from build123d import *

# Parameters (mm, degrees)
SKETCH1_R                         = 4
EXTRUDE1_DEPTH                    = 400
SKETCH3_W                         = 2
SKETCH3_H                         = 4
F_4_0_4_DIAMETER_HOLE1_AT_2_COUNT = 2
F_4_0_4_DIAMETER_HOLE1_AT_2_PITCH = 380


with BuildPart() as part:
    # Sketch1 → Extrude1 (new body)
    with BuildSketch(Plane.XY):
        Circle(SKETCH1_R)
    extrude(amount=EXTRUDE1_DEPTH)

    # Sketch3 → Ø4.0 (4) Diameter Hole1 (revolve, cut)
    with BuildSketch(Plane(origin=(0, 0, 10), x_dir=(0, 0, -1), z_dir=(1, 0, 0))):
        with Locations((1, 2)):
            Rectangle(SKETCH3_W, SKETCH3_H)
    f_4_0_4_diameter_hole1 = revolve(axis=Axis((0, -6.35, 10), (0, 1, 0)), mode=Mode.SUBTRACT)

    # Ø4.0 (4) Diameter Hole1 at 2: Ø4.0 (4) Diameter Hole1 ×2
    with Locations(*[(0, 0, i * F_4_0_4_DIAMETER_HOLE1_AT_2_PITCH) for i in range(1, F_4_0_4_DIAMETER_HOLE1_AT_2_COUNT)]):
        add(f_4_0_4_diameter_hole1, mode=Mode.SUBTRACT)


solid = part.part
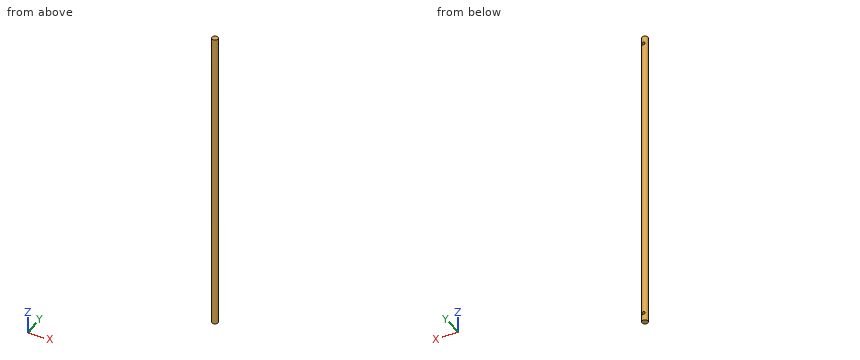
Work out the finished part from the listing and answer in its coordinate system (mm). Give positions to 0.01 mm unless a question says otherwise; leave off trailing zeros. Order: outer loops, then holes, each group sorted by start corner. A loop starts at its lowest first (then second) coordinate and runs counter-clockwise, first axis right, second up. Notation, with made-up numbers: (8, 30.25) -> (21, 30.25) arc R19 ccw to (21, 51.25) -> close; hole circle Ø6 at (-33.5, 59.5). An arc over 180 degrees is marked (long way). Answer as a JSON object with one key per item and string values. Group by question number.
1. Flat-ended cylindrical pins translate along their axes: pin 1 Ø3.5 at (x, z) = (0, 10) entering from +Y; pin 2 Ø1.5 at (y, z) = (-2.5, 178) entering from +X. Find the tip coordinate at first contact, or state that the pin passes through.
2. Consider line 1 along Z through (x, y) = (0.25, 3.75); line 2 along Y through (x, z) = (-0.75, 112); line 3 along X through (y, z) = (1.6, 390). Determine where each line is inside the solid, lowest interval first. Write a range as [from, to].
3. Section A-A on y = 2 is taken. Determine the outline of the cut face in (x, z).
4. Section B-B on z = 140.5 is taken. Determine the outline of the cut face in (x, y), plus the area to 3 significant figures.
Result sheet:
{
 "1": {"pin 1": "stops at y = 0", "pin 2": "stops at x = 3.6"},
 "2": {"line 1": "z = [0, 8.02], [11.98, 388.02], [391.98, 400]", "line 2": "y = [-3.93, 3.93]", "line 3": "x = [-3.67, -2], [2, 3.67]"},
 "3": {"outline": "(-3.46, 0) -> (3.46, 0) -> (3.46, 400) -> (-3.46, 400) -> close; hole circle Ø4 at (0, 10); hole circle Ø4 at (0, 390)"},
 "4": {"outline": "circle Ø8 at (0, 0)", "area": "50.3 mm^2"}
}
